from build123d import *

# Parameters (mm, degrees)
BODY_DEPTH           = 14
TOP_FILLET_R         = 20
SIDE_FILLETS_R       = 2
DESIGN_CHAMFERS_SIZE = 1


# Read off the part's stored shape, not the designer's step: mounting_holes
with BuildPart() as part:
    # Sketch1 → body (new body)
    with BuildSketch(Plane.XY):
        Polygon((0, 0), (88, 0), (88, 10), (74, 10), (64, 30), (64, 50), (24, 50), (24, 30), (14, 10), (0, 10), align=None)
    extrude(amount=BODY_DEPTH)

    # top_fillet
    top_fillet_edges = [part.edges().sort_by_distance(p)[0] for p in [
        (24, 50, 7),
        (64, 50, 7),
    ]]
    fillet(top_fillet_edges, radius=TOP_FILLET_R - 0.0001)  # a hair under: the kernel refuses the full size

    # Sketch4 → bearing_hole (revolve, cut)
    with BuildSketch(Plane(origin=(44, 30, 14), x_dir=(0, -1, 0), z_dir=(1, 0, 0))):
        Polygon((0, 0), (0, 14), (12, 14), (12, 8), (14, 8), (14, 0.5), (14.5, 0), align=None)
    revolve(axis=Axis((44, 30, 20.35), (0, 0, -1)), mode=Mode.SUBTRACT)

    # mounting_holes outline → mounting_holes (revolve, cut)
    with BuildSketch(Plane(origin=(81, 0, 7), x_dir=(1, 0, 0), z_dir=(0, 0, 1))):
        Polygon((0, 0), (2.25, 0), (2.25, 5.6), (4, 5.6), (4, 9.975), (4.025, 10), (0, 10), align=None)
    revolve(axis=Axis((81, 0, 7), (0, 1, 0)), mode=Mode.SUBTRACT)

    # mounting_holes 2 outline → mounting_holes 2 (revolve, cut)
    with BuildSketch(Plane(origin=(7, 0, 7), x_dir=(1, 0, 0), z_dir=(0, 0, 1))):
        Polygon((0, 10), (0, 0), (2.25, 0), (2.25, 5.6), (4, 5.6), (4, 9.975), (4.025, 10), align=None)
    revolve(axis=Axis((7, 0, 7), (0, 1, 0)), mode=Mode.SUBTRACT)

    # side_fillets
    side_fillets_edges = [part.edges().sort_by_distance(p)[0] for p in [
        (88, 5, 14),
        (88, 5, 0),
        (0, 5, 0),
        (0, 5, 14),
    ]]
    fillet(side_fillets_edges, radius=SIDE_FILLETS_R)

    # design_chamfers
    design_chamfers_edges = [part.edges().sort_by_distance(p)[0] for p in [
        (8, 10, 0),
        (19, 20, 0),
        (69, 20, 0),
        (69, 20, 14),
        (58.142164913, 44.142164913, 0),
        (29.857835087, 44.142164913, 0),
        (58.142164913, 44.142164913, 14),
        (29.857835087, 44.142164913, 14),
        (19, 20, 14),
        (8, 10, 14),
        (0, 10, 7),
        (80, 10, 0),
        (0.585786438, 10, 13.414213562),
        (0.585786438, 10, 0.585786438),
        (88, 10, 7),
        (80, 10, 14),
        (87.414213562, 10, 13.414213562),
        (87.414213562, 10, 0.585786438),
    ]]
    chamfer(design_chamfers_edges, length=DESIGN_CHAMFERS_SIZE)


solid = part.part
Input: part model. Units: mm. Frame: model coordinates. A direction names the side the tool comes from. Coordinates: 2 decimals unless noted, no trailing zeros. Order: outer loops, then holes, each group sorted by start corner. A loop starts at its lowest first (then second) coordinate and runs counter-clockwise, first axis right, second up.
1. Contact query for flat-ended pins moving along their axis: P1, Ø3.5, axis at x = 7, z = 7, coming from the -Y side; P2, Ø1.5, axis at x = 79, z = 3.5, coming from the +Y side; P3, Ø2.5, axis at x = 7.5, z = 5, coming from the +Y side. Output: stop coordinate, or through.
Checked values:
P1: passes through
P2: stops at y = 10
P3: stops at y = 5.6
2. Access query for faces 1 (the cylindrical face through (43.384, 43.986, 9.802)), 2 (the cylindrical face through (3.8, 7.8, 9.4)), 3 (the flat face through (19.428, 19.754, 0.507)). Directions: +Z, -Z, +X, -X, +Y, -Y. A direction counts if a zero-diameter tool reaches every point of the face in a straight line with its end or side. Return the directions, or none.
Checked values:
face 1: +Z
face 2: +Y
face 3: -Z, -X, +Y
3. Cut plane B-B, the plane y = 8. Return loops of the section in (x, z), plus the area to 3 significant figures.
Checked values:
outline: (0, 2) arc R2 ccw to (2, 0) - (86, 0) arc R2 ccw to (88, 2) - (88, 12) arc R2 ccw to (86, 14) - (2, 14) arc R2 ccw to (0, 12) - close; hole circle Ø8 at (7, 7); hole circle Ø8 at (81, 7)
area: 1,130 mm2
4. Cut plane C-C, the plane z = 7. Count the separate pieces of the cut face and the enclosed holes in it, plus the area to 3 significant figures.
Checked values:
separate pieces: 3
enclosed holes: 1
area: 1,770 mm2
5. Cut plane A-A, the plane x = 81. Return loops of the section in (y, z) (3 decimals), plus the area to 3 significant figures.
Checked values:
outline: (0, 0) - (9, 0) - (10, 1) - (10, 2.975) - (9.975, 3) - (5.6, 3) - (5.6, 4.75) - (0, 4.75) - close; (0, 9.25) - (5.6, 9.25) - (5.6, 11) - (9.975, 11) - (10, 11.025) - (10, 13) - (9, 14) - (0, 14) - close
area: 78.6 mm2
6. Draft query along X for faces 4 (the flat face through (0, 5, 7)), 5 (the cylindrical face through (83.146, 2.839, 6.324)), 6 (the flat face through (88, 4, 7)). Return one class per face: +X half, -X half, draft (parallel to the pull), parting line (faces both ways), or undercut.
Checked values:
face 4: -X half
face 5: undercut
face 6: +X half
7. Ray query, line 1 along X through (y, z) = (3.65, 7); line 2 along X through (y, z) = (7.1, 7); line 3 along Z through (x, y) = (7, 8). Return the intervals inside material, ascending.
Checked values:
line 1: x = 0 to 4.75, 9.25 to 78.75, 83.25 to 88
line 2: x = 0 to 3, 11 to 77, 85 to 88
line 3: z = 0 to 3, 11 to 14
